Read the model definition and answer for the solid it produces. Units are mm, in the model's axes. Give positions to 0.01 mm unless a question says otherwise; leave off trailing zeros. Write each loop counter-clockwise with the first axis right and the second up, starting at its lowest first coordinate (ties: lowest second). Pieces come first, ordered by that corner, then holes. Notation, with made-up numbers: M 72,54.25 L 93,54.25 A28 ccw 93,72.25 Z; hole C -37.5,-38.5 d7. An arc over 180 degrees is marked long. Use a Markdown table: item, result. Add a question column.
Item 1: Given P1, Ø6, axis at x = 249, z = 132, coming from the -Y side, flat-ended and moving along its own axis, determine where the tip first touches the part or whether it passes through.
Item 2: The mould has two halves that part along X. Classify faces 1 (the flat face through (355.556, 53, 79)), 2 (the flat face through (160, 54, 160)), 3 (the cylindrical face through (-21.948, 9.233, 78.88)): pulls with the +X half, pulls with the -X half, needs draft (parallel to the pull), parting line crosses it, or undercut.
Item 3: Consider probe 1 along X at (y, z) = (77.5, 138.5); probe 2 along X at (y, z) = (15, 84). Determine where each line is inside the solid, lowest interval first. Write a range as [from, to].
Item 4: A cutting plane is placed at A-A on y = 10.5. Determine the outline of the cut face in (x, z).
from build123d import *

# Parameters (mm, degrees)
AUFSATZ_LINEAR_AUSTRAGEN1_DEPTH = 160


with BuildPart() as part:
    # Skizze1 → Aufsatz-Linear austragen1 (new body)
    with BuildSketch(Plane.XY):
        with BuildLine():
            Line((0, 0), (355.55555, 0))
            Line((355.55555, 0), (355.55555, 106.666))
            Line((355.55555, 106.666), (0, 106.666))
            ThreePointArc((0, 106.666), (-21.710167252, 97.673354283), (-30.702812969, 75.963187031))
            Line((-30.702812969, 75.963187031), (-30.702812969, 30.702812969))
            ThreePointArc((-30.702812969, 30.702812969), (-21.710167252, 8.992645717), (0, 0))
        make_face()
    extrude(amount=AUFSATZ_LINEAR_AUSTRAGEN1_DEPTH)


solid = part.part
Filled in:
| question | item | result |
|---|---|---|
| 1 | P1 | y = 0 |
| 2 | face 1 | pulls with the +X half |
| 2 | face 2 | needs draft |
| 2 | face 3 | pulls with the -X half |
| 3 | probe 1 | [-30.66, 355.56] |
| 3 | probe 2 | [-26.38, 355.56] |
| 4 | outline | M -23.12,0 L 355.56,0 L 355.56,160 L -23.12,160 Z |
